CAD build for the part. Positions are in the model's coordinates, mm. A direction names the side the tool comes from. Coordinates: 2 decimals unless noted, no trailing zeros. Write each loop counter-clockwise with the first axis right and the second up, starting at its lowest first coordinate (ties: lowest second). Pieces come first, ordered by that corner, then holes. Notation, with made-up numbers: (71.5, 71.5) - (102.5, 71.5) arc R28 ccw to (102.5, 97.5) - close; hole circle Ø10 at (-22, 65). An arc over 180 degrees is marked (long way). Answer in a Markdown table with one row per item. Add a question column.
Q1. Band-saw the part on C-C (y = 0.4). State how many separate pieces and enclosed holes the cut face has, and give its area (3 significant figures).
Q2. Pin check, flat tips, straight feed: pin 1 (12 mm diameter, centred on x = 4.5, z = 5, fed in from -Y); pin 2 (3 mm diameter, centred on x = 2, z = -2, fed in from +Y); pin 3 (0.8 mm diameter, centred on x = -7.5, y = 0.5, fed in from +Z). Stop position of each tip, or through.
Q3. 3-axis set-ups, long thin cutter, end or side, ignore diameter. For faces 1 (the flat face through (-9.4, 0.5, -3.5)), 2 (the cylindrical face through (-4.672, 0.507, 9.025)), 3 (the flat face through (9.4, 0.5, -3.5)): which of +Z, -Z, +X, -X, +Y, -Y reach the whole face in a straight line?
Q4. Two-plate mould, pull along Z, no slides. Class faces 4 (the flat face through (2.9, 0.5, 9.468)), 5 (the flat face through (4.82, 0.51, -10.29)), 6 (the flat face through (10, 0.5, 4.4)): +Z half, -Z half, draft (parallel to the pull), parting line (faces both ways), or undercut.
Q5. Band-saw the part on B-B (x = 6.25). List the corners of the cut face in (y, z).
Q6. Drill centre lines: line 1 along Z through (x, y) = (-7.75, 0.45); line 2 along X through (y, z) = (0.8, 2.5); line 3 along X through (y, z) = (0.7, 1.75). Where is each one in solid material? Low to high. Write a range as from..to.
Q7. Band-saw the part on A-A (z = 7). List the corners of the cut face in (x, y).
```python
from build123d import *

# Parameters (mm, degrees)
SKETCH1_W            = 20
SKETCH1_H            = 22
BOSS_EXTRUDE1_DEPTH  = 1
CUT_EXTRUDE1_DEPTH   = 2
CUT_EXTRUDE2_DEPTH   = 2
LPATTERN1_COUNT      = 4
LPATTERN1_PITCH      = 4.7
CUT_EXTRUDE3_DEPTH   = 2
SKETCH4_W            = 8.370709726
SKETCH4_H            = 3.642153613
BOSS_EXTRUDE2_DEPTH  = 1.5
SKETCH5_W            = 8.170709726
SKETCH5_H            = 1.3
CUT_EXTRUDE4_DEPTH   = 3.3
CUT_EXTRUDE5_DEPTH   = 1
FILLET1_R            = 0.2
SKETCH7_R            = 0.567557538
CUT_EXTRUDE6_DEPTH   = 1
LPATTERN2_COUNT      = 4
LPATTERN2_PITCH      = 4.7
LPATTERN2_COUNT_DIR2 = 2
LPATTERN2_PITCH_DIR2 = 15.5
BOSS_EXTRUDE3_DEPTH  = 1
FILLET2_R            = 0.8
SKETCH10_W           = 0.699156063
SKETCH10_H           = 0.898914939
CUT_EXTRUDE14_DEPTH  = 11


with BuildPart() as part:
    # Sketch1 → Boss-Extrude1 (new body)
    with BuildSketch(Plane(origin=(0, 0, 0), x_dir=(1, 0, 0), z_dir=(0, 1, 0))):
        Rectangle(SKETCH1_W, SKETCH1_H)
    extrude(amount=BOSS_EXTRUDE1_DEPTH)

    # Sketch2 → Cut-Extrude1 (cut)
    with BuildSketch(Plane(origin=(0, 1, 0), x_dir=(1, 0, 0), z_dir=(0, 1, 0))):
        Polygon((-10, -11), (-3.81466663, -11), (-5.992999925, -9.366600626), (-9.260499866, -9.366600626), (-10, -8.38038881), align=None)
        Polygon((5.992999925, -9.366600626), (3.81466663, -11), (10, -11), (10, -8.38038881), (9.260499866, -9.366600626), align=None)
    extrude(amount=-CUT_EXTRUDE1_DEPTH, mode=Mode.SUBTRACT)

    # Sketch2_3 → Cut-Extrude2 (cut)
    with BuildSketch(Plane(origin=(0, 1, 0), x_dir=(1, 0, 0), z_dir=(0, 1, 0))):
        Polygon((-10, -5.098741352), (-10, -8.38038881), (-8.769646289, -6.739565081), align=None)
        Polygon((8.769646289, -6.739565081), (10, -8.38038881), (10, -5.098741352), align=None)
    cut_extrude2 = extrude(amount=-CUT_EXTRUDE2_DEPTH, mode=Mode.SUBTRACT)

    # LPattern1: Cut-Extrude2 ×4
    with Locations(*[(0, 0, -i * LPATTERN1_PITCH) for i in range(1, LPATTERN1_COUNT)]):
        add(cut_extrude2, mode=Mode.SUBTRACT)

    # Sketch3 → Cut-Extrude3 (cut)
    with BuildSketch(Plane(origin=(0, 1, 0), x_dir=(1, 0, 0), z_dir=(0, 1, 0))):
        Polygon((-5.546503539, 9.56506288), (-4.111566419, 11), (-10, 11), (-10, 9.001258648), (-9.436195769, 9.56506288), align=None)
        Polygon((9.436195769, 9.56506288), (10, 9.001258648), (10, 11), (4.111566419, 11), (5.546503539, 9.56506288), align=None)
    extrude(amount=-CUT_EXTRUDE3_DEPTH, mode=Mode.SUBTRACT)

    # Sketch4 → Boss-Extrude2 (add)
    with BuildSketch(Plane(origin=(0, 1, 0), x_dir=(1, 0, 0), z_dir=(0, 1, 0))):
        with Locations((0, 9.105134748)):
            Rectangle(SKETCH4_W, SKETCH4_H)
    extrude(amount=BOSS_EXTRUDE2_DEPTH)

    # Sketch5 → Cut-Extrude4 (cut)
    with BuildSketch(Plane(origin=(0, 0, -10.926211555), x_dir=(-1, 0, 0), z_dir=(0, 0, -1))):
        with Locations((0, 1.75)):
            Rectangle(SKETCH5_W, SKETCH5_H)
    extrude(amount=-CUT_EXTRUDE4_DEPTH, mode=Mode.SUBTRACT)

    # Sketch6 → Cut-Extrude5 (cut)
    with BuildSketch(Plane(origin=(0, 2.5, 0), x_dir=(1, 0, 0), z_dir=(0, 1, 0))):
        with BuildLine():
            Line((-2.493852215, 10.469900747), (-2.493852215, 9.144845176))
            ThreePointArc((-2.493852215, 9.144845176), (-2.733489924, 8.905207467), (-2.973127634, 9.144845176))
            Line((-2.973127634, 9.144845176), (-2.973127634, 10.469900747))
            ThreePointArc((-2.973127634, 10.469900747), (-2.733489924, 10.709538456), (-2.493852215, 10.469900747))
        make_face()
        with BuildLine():
            Line((2.493852215, 10.469900747), (2.493852215, 9.144845176))
            ThreePointArc((2.493852215, 9.144845176), (2.733489924, 8.905207467), (2.973127634, 9.144845176))
            Line((2.973127634, 9.144845176), (2.973127634, 10.469900747))
            ThreePointArc((2.973127634, 10.469900747), (2.733489924, 10.709538456), (2.493852215, 10.469900747))
        make_face()
    extrude(amount=-CUT_EXTRUDE5_DEPTH, mode=Mode.SUBTRACT)

    # Fillet1
    fillet1_edges = [part.edges().sort_by_distance(p)[0] for p in [
        (4.185354863, 2.5, -9.105134749),
        (-4.185354863, 2.5, -9.105134749),
        (0, 2.5, -7.284057942),
    ]]
    fillet(fillet1_edges, radius=FILLET1_R)

    # Sketch7 → Cut-Extrude6 (cut)
    with BuildSketch(Plane(origin=(0, 1, 0), x_dir=(1, 0, 0), z_dir=(0, 1, 0))):
        with Locations(Location((-7.769646289, -6.739565081, 0), (0, 0, 270))):
            Circle(SKETCH7_R)
    cut_extrude6 = extrude(amount=-CUT_EXTRUDE6_DEPTH, mode=Mode.SUBTRACT)

    # LPattern2: Cut-Extrude6 4 × 2
    with Locations(*[(j * LPATTERN2_PITCH_DIR2, 0, -i * LPATTERN2_PITCH) for i in range(LPATTERN2_COUNT) for j in range(LPATTERN2_COUNT_DIR2) if (i, j) != (0, 0)]):
        add(cut_extrude6, mode=Mode.SUBTRACT)

    # Sketch8 → Boss-Extrude3 (add)
    with BuildSketch(Plane(origin=(0, 1, 0), x_dir=(1, 0, 0), z_dir=(0, 1, 0))):
        Polygon((-4.226815495, -0.36610213), (-0.36610213, 4.226815495), (4.226815495, 0.36610213), (0.36610213, -4.226815495), align=None)
    extrude(amount=BOSS_EXTRUDE3_DEPTH)

    # Fillet2
    fillet2_edges = [part.edges().sort_by_distance(p)[0] for p in [
        (-1.930356683, 2, 2.296458812),
        (2.296458812, 2, 1.930356683),
        (1.930356683, 2, -2.296458812),
        (-2.296458812, 2, -1.930356683),
    ]]
    fillet(fillet2_edges, radius=FILLET2_R)

    # Sketch10 → Cut-Extrude14 (cut)
    with BuildSketch(Plane(origin=(0, 2, 0), x_dir=(1, 0, 0), z_dir=(0, 1, 0))):
        with BuildLine():
            Line((-2.425111335, -8.585549508), (-2.974448243, -8.585549508))
            Line((-2.974448243, -8.585549508), (-2.974448243, -9.484464447))
            Line((-2.974448243, -9.484464447), (-2.425111335, -9.484464447))
            ThreePointArc((-2.425111335, -9.484464447), (-1.975653866, -9.035006978), (-2.425111335, -8.585549508))
        make_face()
        with BuildLine():
            Line((-3.673604306, -8.585549508), (-4.222941213, -8.585549508))
            ThreePointArc((-4.222941213, -8.585549508), (-4.672398683, -9.035006978), (-4.222941213, -9.484464447))
            Line((-4.222941213, -9.484464447), (-3.673604306, -9.484464447))
            Line((-3.673604306, -9.484464447), (-3.673604306, -8.585549508))
        make_face()
        with BuildLine():
            Line((-3.673604306, -8.052859174), (-3.673604306, -8.585549508))
            Line((-3.673604306, -8.585549508), (-2.974448243, -8.585549508))
            Line((-2.974448243, -8.585549508), (-2.974448243, -8.052859174))
            ThreePointArc((-2.974448243, -8.052859174), (-3.324026274, -7.703281142), (-3.673604306, -8.052859174))
        make_face()
        with Locations((-3.324026275, -9.035006978)):
            Rectangle(SKETCH10_W, SKETCH10_H)
        with BuildLine():
            Line((-2.974448243, -9.484464447), (-3.673604306, -9.484464447))
            Line((-3.673604306, -9.484464447), (-3.673604306, -10.017154782))
            ThreePointArc((-3.673604306, -10.017154782), (-3.324026274, -10.366732814), (-2.974448243, -10.017154782))
            Line((-2.974448243, -10.017154782), (-2.974448243, -9.484464447))
        make_face()
        with BuildLine():
            Line((2.06946336, -9.467817874), (3.834000092, -9.467817874))
            ThreePointArc((3.834000092, -9.467817874), (4.266810989, -9.035006978), (3.834000092, -8.602196081))
            Line((3.834000092, -8.602196081), (2.06946336, -8.602196081))
            ThreePointArc((2.06946336, -8.602196081), (1.636652464, -9.035006978), (2.06946336, -9.467817874))
        make_face()
    extrude(amount=-CUT_EXTRUDE14_DEPTH, mode=Mode.SUBTRACT)


solid = part.part
```
Checked values:
| question | item | result |
|---|---|---|
| 1 | separate pieces | 1 |
| 1 | enclosed holes | 10 |
| 1 | area | 378 mm² |
| 2 | pin 1 | stops at y = 0 |
| 2 | pin 2 | stops at y = 2 |
| 2 | pin 3 | stops at z = 9.37 |
| 3 | face 1 | -X, +Y, -Y |
| 3 | face 2 | +Y, -Y |
| 3 | face 3 | +X, +Y, -Y |
| 4 | face 4 | undercut |
| 4 | face 5 | -Z half |
| 4 | face 6 | draft |
| 5 | outline | (0, -9.57) - (1, -9.57) - (1, 9.37) - (0, 9.37) - close |
| 6 | line 1 | z = -9.57..-7.93, -6.79..-3.23, -2.09..1.47, 2.61..6.17, 7.31..9.37 |
| 6 | line 2 | x = -9.11..-8.1, -7.44..7.4, 8.06..9.11 |
| 6 | line 3 | x = -8.99..-8.26, -7.28..7.24, 8.22..8.99 |
| 7 | outline | (-8.96, 0) - (-8.27, 0) - (-8.27, 1) - (-8.96, 1) - close; (-7.27, 0) - (7.23, 0) - (7.23, 1) - (-7.27, 1) - close; (8.23, 0) - (8.96, 0) - (8.96, 1) - (8.23, 1) - close |
